```python
from build123d import *

# Parameters (mm, degrees)
SKETCH_W      = 12
SKETCH_H      = 120
SKETCH_W_2    = 6.05
SKETCH_H_2    = 3.05
PAD_DEPTH     = 4
SKETCH001_R   = 1.2
HOLE_DEPTH    = 25
SKETCH002_W   = 10.05
SKETCH002_H   = 4.05
SKETCH002_W_2 = 6.05
SKETCH002_H_2 = 3.05
PAD001_DEPTH  = 2.5
SKETCH003_W   = 10.05
SKETCH003_H   = 4.05
PAD002_DEPTH  = 2
SKETCH004_R   = 2.5
POCKET_DEPTH  = 0.5


with BuildPart() as part:
    # Sketch → Pad (new body)
    with BuildSketch(Plane.XY):
        Rectangle(SKETCH_W, SKETCH_H)
        with Locations((0, 57.975)):
            Rectangle(SKETCH_W_2, SKETCH_H_2, mode=Mode.SUBTRACT)
    extrude(amount=PAD_DEPTH)

    # Sketch001 (on Face10 of Pad) → Hole (cut)
    with BuildSketch(Plane.XY.offset(4)):
        with Locations((3, 54)):
            Circle(SKETCH001_R)
        with Locations((3, 4)):
            Circle(SKETCH001_R)
        with Locations((3, -46)):
            Circle(SKETCH001_R)
        with Locations((-3, 54)):
            Circle(SKETCH001_R)
        with Locations((-3, 4)):
            Circle(SKETCH001_R)
        with Locations((-3, -46)):
            Circle(SKETCH001_R)
    extrude(amount=-HOLE_DEPTH, mode=Mode.SUBTRACT)

    # Sketch002 (on Face5 of Hole) → Pad001 (join)
    with BuildSketch(Plane.XY.offset(4)):
        with Locations((0, 57.975)):
            Rectangle(SKETCH002_W, SKETCH002_H)
        with Locations((0, 57.975)):
            Rectangle(SKETCH002_W_2, SKETCH002_H_2, mode=Mode.SUBTRACT)
    extrude(amount=PAD001_DEPTH)

    # Sketch003 (on Face15 of Pad001) → Pad002 (join)
    with BuildSketch(Plane.XY.offset(6.5)):
        with Locations((0, 57.975)):
            Rectangle(SKETCH003_W, SKETCH003_H)
    extrude(amount=PAD002_DEPTH)

    # Sketch004 (on Face17 of Pad002) → Pocket (cut)
    with BuildSketch(Plane(origin=(0, 60, 0), x_dir=(-1, 0, 0), z_dir=(0, 1, 0))):
        with Locations((0, 3.25)):
            Circle(SKETCH004_R)
    extrude(amount=-POCKET_DEPTH, mode=Mode.SUBTRACT)


solid = part.part
```
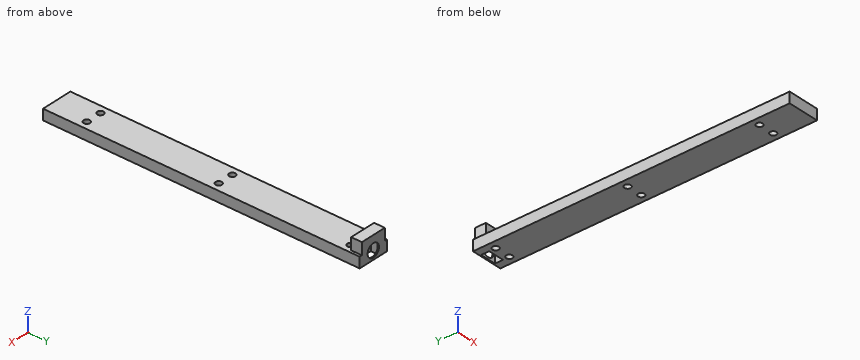
Work out the finished part from the listing and answer in its coordinate system (mm). Give positions to 0.01 mm unless a question says otherwise; leave off trailing zeros. Write each loop counter-clockwise with the first axis right and the second up, starting at its lowest first coordinate (ties: lowest second). Pieces come first, ordered by that corner, then holes. Notation, with made-up numbers: (46, 77.5) -> (51, 77.5) arc R19 ccw to (51, 113.5) -> close; hole circle Ø6 at (-18.75, 52.25). An arc over 180 degrees is marked (long way). Write each question's results on one line, items separated by ' | '.
1. Find section B-B on x = 0.75. Determine the outline of the cut face in (y, z), and give its area (3 significant figures).
Data:
outline: (-60, 0) -> (56.45, 0) -> (56.45, 6.5) -> (59.5, 6.5) -> (59.5, 5.63) -> (60, 5.63) -> (60, 8.5) -> (55.95, 8.5) -> (55.95, 4) -> (-60, 4) -> close; (59.5, 0) -> (60, 0) -> (60, 0.87) -> (59.5, 0.87) -> close | area: 476 mm^2
2. Find section C-C on y = -42.5. Determine the outline of the cut face in (x, z), and give its area (3 significant figures).
Data:
outline: (-6, 0) -> (6, 0) -> (6, 4) -> (-6, 4) -> close | area: 48.0 mm^2
3. Each of these flat-tipped pins is pushed along its axis until it touches: pin 1 Ø3 at (y, z) = (59, 6.5) entering from +X (3 decimals); pin 2 Ø2 at (x, z) = (2.5, 5.5) entering from -Y; pin 3 Ø1.5 at (x, y) = (0, 58.5) entering from -Z. Where does it stop, or does it pass through?
Data:
pin 1: x = 5.025 | pin 2: y = 55.95 | pin 3: z = 6.5
4. Find section A-A on y = 54. Determine the outline of the cut face in (x, z).
Data:
outline: (-6, 0) -> (-4.2, 0) -> (-4.2, 4) -> (-6, 4) -> close; (-1.8, 0) -> (1.8, 0) -> (1.8, 4) -> (-1.8, 4) -> close; (4.2, 0) -> (6, 0) -> (6, 4) -> (4.2, 4) -> close
5. Straight lines are drawn through the part: L1, parallel to Y at x = -4, z = 2.25; L2, parallel to Z at x = -4.75, y = 33; L3, parallel to Y at x = -0.5, z = 3.25. For each, find the intervals that lie inside material, in ascending order.
Data:
L1: -60 to -46.66, -45.34 to 3.34, 4.66 to 53.34, 54.66 to 60 | L2: 0 to 4 | L3: -60 to 56.45
